Input: part model. Units: mm. Frame: model coordinates. A direction names the side the tool comes from. Give positions to 0.01 mm unless a question says otherwise; leave off trailing zeros. Loops run counter-clockwise (first coordinate to the right, second up) from the corner with the lowest first, then second, coordinate; pieces in that order, holes last.
from build123d import *

# Parameters (mm, degrees)
SKETCH_1_W          = 30.7
SKETCH_1_H          = 30.7
EXTRUDE_1_DEPTH     = 26.9
SKETCH_2_R          = 14.5
EXTRUDE_2_DEPTH     = 2.5
SKETCH_3_R          = 9.5
EXTRUDE_3_DEPTH     = 0.5
CHAMFER_1_SIZE      = 0.5
CHAMFER_2_SIZE      = 0.3
SKETCH_4_R          = 4.5
EXTRUDE_4_DEPTH     = 20
SKETCH_5_R          = 8
EXTRUDE_5_DEPTH     = 2.6
SKETCH_6_R          = 2.5
EXTRUDE_6_DEPTH     = 13
CHAMFER_3_SIZE      = 0.5
CUT_EXTRUDE_1_DEPTH = 1.5
SKETCH_8_R          = 1.5
CUT_EXTRUDE_2_DEPTH = 6
SKETCH_9_R          = 1.25
CUT_EXTRUDE_3_DEPTH = 1.5
SKETCH_10_R         = 1.5
CUT_EXTRUDE_4_DEPTH = 4
SKETCH_11_R         = 1.25
CUT_EXTRUDE_5_DEPTH = 1.5
CHAMFER_4_SIZE      = 2.529
CHAMFER_5_SIZE      = 0.5
CUT_EXTRUDE_START   = -18
CUT_EXTRUDE_6_DEPTH = 18
CUT_EXTRUDE_START_2 = -11
CUT_EXTRUDE_7_DEPTH = 11


with BuildPart() as part:
    # 草图1 → 凸台-拉伸1 (new body)
    with BuildSketch(Plane(origin=(0, 0, 0), x_dir=(1, 0, 0), z_dir=(0, 1, 0))):
        Rectangle(SKETCH_1_W, SKETCH_1_H)
    extrude(amount=EXTRUDE_1_DEPTH)

    # 草图2 → 凸台-拉伸2 (add)
    with BuildSketch(Plane(origin=(0, 26.9, 0), x_dir=(1, 0, 0), z_dir=(0, 1, 0))):
        with Locations(Location((0, 0, 0), (0, 0, 270))):
            Circle(SKETCH_2_R)
    extrude(amount=EXTRUDE_2_DEPTH)

    # 草图3 → 凸台-拉伸3 (add)
    with BuildSketch(Plane(origin=(0, 29.4, 0), x_dir=(1, 0, 0), z_dir=(0, 1, 0))):
        with Locations(Location((0, 0, 0), (0, 0, 270))):
            Circle(SKETCH_3_R)
    extrude(amount=EXTRUDE_3_DEPTH)

    # 倒角1
    chamfer_1_edges = [part.edges().sort_by_distance(p)[0] for p in [
        (0, 29.4, -9.5),
    ]]
    chamfer(chamfer_1_edges, length=CHAMFER_1_SIZE - 0.0001)  # a hair under: the kernel refuses the full size

    # 倒角2
    chamfer_2_edges = [part.edges().sort_by_distance(p)[0] for p in [
        (0, 29.4, -14.5),
    ]]
    chamfer(chamfer_2_edges, length=CHAMFER_2_SIZE)

    # 草图4 → 凸台-拉伸4 (add)
    with BuildSketch(Plane(origin=(0, 29.9, 0), x_dir=(1, 0, 0), z_dir=(0, 1, 0))):
        with Locations(Location((0, 0, 0), (0, 0, 270))):
            Circle(SKETCH_4_R)
    extrude(amount=EXTRUDE_4_DEPTH)

    # 草图5 → 凸台-拉伸5 (add)
    with BuildSketch(Plane.XZ):
        with Locations(Location((0, 0, 0), (0, 0, 270))):
            Circle(SKETCH_5_R)
    extrude(amount=EXTRUDE_5_DEPTH)

    # 草图6 → 凸台-拉伸6 (add)
    with BuildSketch(Plane.XZ.offset(2.6)):
        with Locations(Location((0, 0, 0), (0, 0, 90))):
            Circle(SKETCH_6_R)
    extrude(amount=EXTRUDE_6_DEPTH)

    # 倒角3
    chamfer_3_edges = [part.edges().sort_by_distance(p)[0] for p in [
        (0, -2.6, 8),
        (0, -15.6, -2.5),
    ]]
    chamfer(chamfer_3_edges, length=CHAMFER_3_SIZE)

    # 草图7 → 切除-拉伸1 (cut)
    with BuildSketch(Plane.XZ):
        with BuildLine():
            Line((-15.35, 8.75), (-12, 8.75))
            ThreePointArc((-12, 8.75), (-9.701902961, 9.701902961), (-8.75, 12))
            Line((-8.75, 12), (-8.75, 15.35))
            Line((-8.75, 15.35), (-15.35, 15.35))
            Line((-15.35, 15.35), (-15.35, 8.75))
        make_face()
        with BuildLine():
            Line((15.35, -15.35), (15.35, -8.75))
            Line((15.35, -8.75), (12, -8.75))
            ThreePointArc((12, -8.75), (9.701902961, -9.701902961), (8.75, -12))
            Line((8.75, -12), (8.75, -15.35))
            Line((8.75, -15.35), (15.35, -15.35))
        make_face()
    extrude(amount=-CUT_EXTRUDE_1_DEPTH, mode=Mode.SUBTRACT)

    # 草图8 → 切除-拉伸2 (cut)
    with BuildSketch(Plane(origin=(0, 26.9, 0), x_dir=(1, 0, 0), z_dir=(0, 1, 0))):
        with Locations(Location((-12.374368671, 12.374368671, 0), (0, 0, 270))):
            Circle(SKETCH_8_R)
        with Locations(Location((12.374368671, 12.374368671, 0), (0, 0, 270))):
            Circle(SKETCH_8_R)
        with Locations(Location((12.374368671, -12.374368671, 0), (0, 0, 270))):
            Circle(SKETCH_8_R)
        with Locations(Location((-12.374368671, -12.374368671, 0), (0, 0, 270))):
            Circle(SKETCH_8_R)
    extrude(amount=-CUT_EXTRUDE_2_DEPTH, mode=Mode.SUBTRACT)

    # 草图9 → 切除-拉伸3 (cut)
    with BuildSketch(Plane(origin=(0, 20.9, 0), x_dir=(1, 0, 0), z_dir=(0, 1, 0))):
        with Locations(Location((12.374368671, -12.374368671, 0), (0, 0, 270))):
            Circle(SKETCH_9_R)
        with Locations(Location((12.374368671, 12.374368671, 0), (0, 0, 270))):
            Circle(SKETCH_9_R)
        with Locations(Location((-12.374368671, 12.374368671, 0), (0, 0, 270))):
            Circle(SKETCH_9_R)
        with Locations(Location((-12.374368671, -12.374368671, 0), (0, 0, 270))):
            Circle(SKETCH_9_R)
    extrude(amount=-CUT_EXTRUDE_3_DEPTH, mode=Mode.SUBTRACT)

    # 草图10 → 切除-拉伸4 (cut)
    with BuildSketch(Plane(origin=(0, 29.9, 0), x_dir=(1, 0, 0), z_dir=(0, 1, 0))):
        with Locations(Location((-7.75, 0, 0), (0, 0, 270))):
            Circle(SKETCH_10_R)
        with Locations(Location((0, 7.75, 0), (0, 0, 270))):
            Circle(SKETCH_10_R)
        with Locations(Location((7.75, 0, 0), (0, 0, 270))):
            Circle(SKETCH_10_R)
        with Locations(Location((0, -7.75, 0), (0, 0, 270))):
            Circle(SKETCH_10_R)
    extrude(amount=-CUT_EXTRUDE_4_DEPTH, mode=Mode.SUBTRACT)

    # 草图11 → 切除-拉伸5 (cut)
    with BuildSketch(Plane(origin=(0, 25.9, 0), x_dir=(1, 0, 0), z_dir=(0, 1, 0))):
        with Locations(Location((0, 7.75, 0), (0, 0, 270))):
            Circle(SKETCH_11_R)
        with Locations(Location((-7.75, 0, 0), (0, 0, 270))):
            Circle(SKETCH_11_R)
        with Locations(Location((7.75, 0, 0), (0, 0, 270))):
            Circle(SKETCH_11_R)
        with Locations(Location((0, -7.75, 0), (0, 0, 270))):
            Circle(SKETCH_11_R)
    extrude(amount=-CUT_EXTRUDE_5_DEPTH, mode=Mode.SUBTRACT)

    # 倒角4
    chamfer_4_edges = [part.edges().sort_by_distance(p)[0] for p in [
        (-15.35, 13.45, -15.35),
        (15.35, 14.2, -15.35),
        (15.35, 13.45, 15.35),
        (-15.35, 14.2, 15.35),
    ]]
    chamfer(chamfer_4_edges, length=CHAMFER_4_SIZE)

    # 倒角5
    chamfer_5_edges = [part.edges().sort_by_distance(p)[0] for p in [
        (0, 49.9, -4.5),
    ]]
    chamfer(chamfer_5_edges, length=CHAMFER_5_SIZE)

    # 草图12 → 切除-拉伸6 (cut)
    with BuildSketch(Plane(origin=(0, 49.9, 0), x_dir=(1, 0, 0), z_dir=(0, 1, 0)).offset(CUT_EXTRUDE_START)):
        with BuildLine():
            Line((-2.828427125, 3.5), (2.828427125, 3.5))
            ThreePointArc((2.828427125, 3.5), (0, 4.5), (-2.828427125, 3.5))
        make_face()
    extrude(amount=CUT_EXTRUDE_6_DEPTH, mode=Mode.SUBTRACT)

    # 草图13 → 切除-拉伸7 (cut)
    with BuildSketch(Plane.XZ.offset(15.6).offset(CUT_EXTRUDE_START_2)):
        with BuildLine():
            Line((-1.5, -2), (1.5, -2))
            ThreePointArc((1.5, -2), (0, -2.5), (-1.5, -2))
        make_face()
    extrude(amount=CUT_EXTRUDE_7_DEPTH, mode=Mode.SUBTRACT)


solid = part.part
(1) Cut plane A-A (y = -5.5). Return the cut outline in (x, z).
Values follow:
outline: (-1.5, -2) - (1.5, -2) arc R2.5 ccw (long way) to start
(2) Pin query (flat end, axial travel): pin 1 Ø1.2 at (x, z) = (12, -13) entering from +Y; pin 2 Ø0.9 at (x, z) = (-0.5, 7.5) entering from +Y; pin 3 Ø2 at (x, z) = (-7.5, -0.5) entering from +Y. Return the tip coordinate at first contact, or that it passes through.
Values follow:
pin 1: stops at y = 20.9
pin 2: stops at y = 24.4
pin 3: stops at y = 29.9
(3) Ray query, probe 1 along X at (y, z) = (25, 0); probe 2 along X at (y, z) = (27.35, 0); probe 3 along Y at (x, z) = (13, -8). Return the intervals inside material, ascending.
Values follow:
probe 1: x = -15.35 to -9, -6.5 to 6.5, 9 to 15.35
probe 2: x = -14.5 to -9.25, -6.25 to 6.25, 9.25 to 14.5
probe 3: y = 0 to 26.9
(4) Reachability of faces 5 (the cylindrical face through (-11.32, 20.16, -11.7)), 6 (the cylindrical face through (-9.727, 0.74, 9.677)), 7 (the flat face through (8.75, 1, -14)), 8 (the flat face through (7, 0, -7)) from +Z, -Z, +X, -X, +Y, -Y: full face, straight path, thin tool, end or side. Return the list, or none.
Values follow:
face 5: +Y
face 6: +Z, -X, -Y
face 7: -Z, +X, -Y
face 8: -Y
(5) Mould query, pull axis Z, two halves, no side actions, for faces 1 (the flat face through (14.07, 13.26, 14.1)), 2 (the cylindrical face through (11.9, 20.16, 13.53)), 3 (the flat face through (14.1, 14.02, -14.07)), 4 (the flat face through (0, 49.9, 0)). Classes: +Z half, -Z half, draft (parallel to the pull), parting line (faces both ways), or undercut.
Values follow:
face 1: +Z half
face 2: undercut
face 3: -Z half
face 4: draft
